Answer from the drawing. Dimensions are ordinates in mm from the lowest x, y and z of the part. Coordinates: 2 decimals unless noted, no trailing zeros. Order: outer loops, then holes, each group sorted by start corner. A loop starts at its lowest first (then second) coordinate and runs counter-clockwise, first axis right, second up. Notation, with made-up numbers: M -23,-22 L 29,-22 A16 ccw 29,-5 Z; hole C -2.5,27.5 d8. An arc over 180 degrees is marked long. Use a Markdown table: item, result.
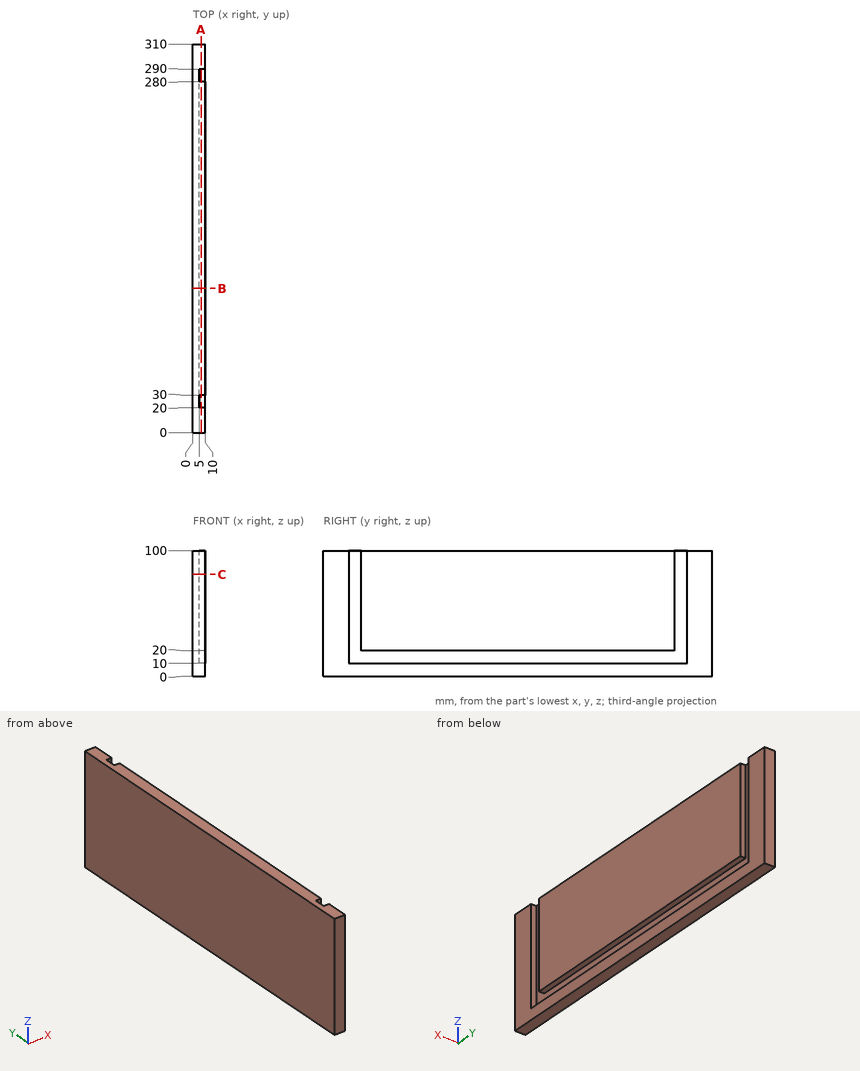
(1) Straight lines are drawn through the part: L1, parallel to Y at x = 5.5, z = 58; L2, parallel to Z at x = 6.75, y = 156; L3, parallel to X at y = 146.5, z = 17.5. For each, find the intervals that lie inside material, in ascending order.
Conclusion:
| item | result |
|---|---|
| L1 | 0 to 20, 30 to 280, 290 to 310 |
| L2 | 0 to 10, 20 to 100 |
| L3 | 0 to 5 |
(2) A cutting plane is placed at B-B (y = 115). Determine the outline of the cut face in (x, z), then the cut area to 3 significant figures.
Conclusion:
| item | result |
|---|---|
| outline | M 0,0 L 10,0 L 10,10 L 5,10 L 5,20 L 10,20 L 10,100 L 0,100 Z |
| area | 950 mm2 |
(3) A cutting plane is placed at A-A (x = 6.5). Determine the outline of the cut face in (y, z).
Conclusion:
| item | result |
|---|---|
| outline | M 0,0 L 310,0 L 310,100 L 290,100 L 290,10 L 20,10 L 20,100 L 0,100 Z; M 30,20 L 280,20 L 280,100 L 30,100 Z |
(4) Given P1, Ø4, axis at x = 7, y = 143, coming from the -Z side, flat-ended and moving along its own axis, determine where the tip first touches the part or whether it passes through.
Conclusion:
| item | result |
|---|---|
| P1 | z = 0 |
(5) A cutting plane is placed at C-C (z = 81). Determine the outline of the cut face in (x, y).
Conclusion:
| item | result |
|---|---|
| outline | M 0,0 L 10,0 L 10,20 L 5,20 L 5,30 L 10,30 L 10,280 L 5,280 L 5,290 L 10,290 L 10,310 L 0,310 Z |
